Work out the finished part from the listing and answer in its coordinate system (mm). Face numbers are marked on the shaded views. A direction names the side the tool comes from. Coordinates: 2 decimals unless noted, no trailing zeros. Write each loop counter-clockwise with the first axis right and the second up, starting at its lowest first coordinate (ties: lowest second). Pieces come first, ordered by that corner, then holes. Notation, with made-up numbers: (-38.75, 59.5) - (-32.75, 59.5) arc R22 cw to (-32.75, 74.5) - close; hole circle Ø5 at (-15, 43.5). An arc over 180 degrees is marked (long way). Use a Markdown table: item, result. Add a question column.
(1) A tool of negligible diameter and unlimited length cuts with its end or side. For the marked faces 5 and 6, from which of +Z, -Z, +X, -X, +Y, -Y can it reach the whole face along a straight path? Write none if from no direction.
(2) For a pull along X with two mould halves and no side action, classify the marked faces 1, 2, 3 and 4 as released by +X, released by -X, zero draft, split by the parting line, or undercut.
(3) Find the intervals of material crossed by line 1 (X direction, y = 7.95, z = -20); line 2 (Z direction, x = 32, y = 3.2); line 3 (X direction, y = 3.4, z = 20), in increasing order. Write a range as from..to.
(4) The part is cut by section A-A, the plane z = 20. Give the vertices of the cut face in (x, y).
(5) Given pin 1 Ø6 at (x, z) = (-28.5, -5.5) entering from +Y; pin 2 Ø6.5 at (x, z) = (30.5, 20.5) entering from +Y; pin 3 Ø4 at (x, z) = (32, 20) entering from +Y, each flat-ended and moving along its own axis, determine where each tip first touches the part or whether it passes through.
(6) The part is cut by section C-C, the plane y = 35. Give the vertices of the cut face in (x, z).
(7) The part is cut by section B-B, the plane z = 2. Give the vertices of the cut face in (x, y).
(8) The part is cut by section D-D, the plane z = -20. Give the vertices of the cut face in (x, y), then the cut area to 3 significant figures.
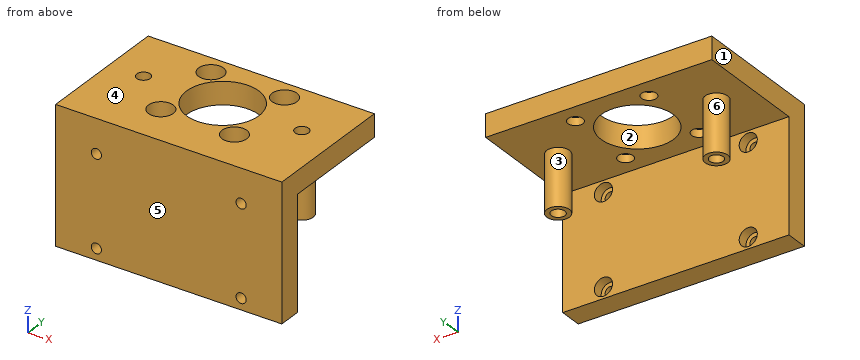
from build123d import *

# Parameters (mm, degrees)
SKETCH1_W           = 100
SKETCH1_H           = 50
BOSS_EXTRUDE1_DEPTH = 10
SKETCH2_R           = 2.25
CUT_EXTRUDE1_DEPTH  = 11
SKETCH3_R           = 4
CUT_EXTRUDE2_DEPTH  = 4.4
SKETCH4_W           = 100
SKETCH4_H           = 60
BOSS_EXTRUDE2_DEPTH = 10
SKETCH5_R           = 16
CUT_EXTRUDE3_DEPTH  = 11
SKETCH6_R           = 3.3
CUT_EXTRUDE4_DEPTH  = 11
SKETCH7_R           = 5.5
CUT_EXTRUDE5_DEPTH  = 6.6
SKETCH8_R           = 3
CUT_EXTRUDE6_DEPTH  = 11
SKETCH9_R           = 5
SKETCH9_R_2         = 3
BOSS_EXTRUDE3_DEPTH = 25


with BuildPart() as part:
    # Sketch1 → Boss-Extrude1 (new body)
    with BuildSketch(Plane(origin=(0, 0, 0), x_dir=(1, 0, 0), z_dir=(0, 1, 0))):
        Rectangle(SKETCH1_W, SKETCH1_H)
    extrude(amount=BOSS_EXTRUDE1_DEPTH)

    # Sketch2 → Cut-Extrude1 (cut, through all)
    with BuildSketch(Plane(origin=(0, 10, 0), x_dir=(1, 0, 0), z_dir=(0, 1, 0))):
        with Locations((32, 20)):
            Circle(SKETCH2_R)
        with Locations((32, -20)):
            Circle(SKETCH2_R)
        with Locations((-32, 20)):
            Circle(SKETCH2_R)
        with Locations((-32, -20)):
            Circle(SKETCH2_R)
    extrude(amount=-CUT_EXTRUDE1_DEPTH, mode=Mode.SUBTRACT)

    # Sketch3 → Cut-Extrude2 (cut)
    with BuildSketch(Plane(origin=(0, 10, 0), x_dir=(1, 0, 0), z_dir=(0, 1, 0))):
        with Locations((32, 20)):
            Circle(SKETCH3_R)
        with Locations((32, -20)):
            Circle(SKETCH3_R)
        with Locations((-32, 20)):
            Circle(SKETCH3_R)
        with Locations((-32, -20)):
            Circle(SKETCH3_R)
    extrude(amount=-CUT_EXTRUDE2_DEPTH, mode=Mode.SUBTRACT)

    # Sketch4 → Boss-Extrude2 (add)
    with BuildSketch(Plane.XY.offset(25)):
        with Locations((0, 30)):
            Rectangle(SKETCH4_W, SKETCH4_H)
    extrude(amount=BOSS_EXTRUDE2_DEPTH)

    # Sketch5 → Cut-Extrude3 (cut, through all)
    with BuildSketch(Plane(origin=(0, 0, 25), x_dir=(-1, 0, 0), z_dir=(0, 0, -1))):
        with Locations((0, 35)):
            Circle(SKETCH5_R)
    extrude(amount=-CUT_EXTRUDE3_DEPTH, mode=Mode.SUBTRACT)

    # Sketch6 → Cut-Extrude4 (cut, through all)
    with BuildSketch(Plane(origin=(0, 0, 25), x_dir=(-1, 0, 0), z_dir=(0, 0, -1))):
        with Locations((-16.25, 51.25)):
            Circle(SKETCH6_R)
        with Locations((-16.25, 18.75)):
            Circle(SKETCH6_R)
        with Locations((16.25, 18.75)):
            Circle(SKETCH6_R)
        with Locations((16.25, 51.25)):
            Circle(SKETCH6_R)
    extrude(amount=-CUT_EXTRUDE4_DEPTH, mode=Mode.SUBTRACT)

    # Sketch7 → Cut-Extrude5 (cut)
    with BuildSketch(Plane.XY.offset(35)):
        with Locations((-16.25, 51.25)):
            Circle(SKETCH7_R)
        with Locations((16.25, 51.25)):
            Circle(SKETCH7_R)
        with Locations((16.25, 18.75)):
            Circle(SKETCH7_R)
        with Locations((-16.25, 18.75)):
            Circle(SKETCH7_R)
    extrude(amount=-CUT_EXTRUDE5_DEPTH, mode=Mode.SUBTRACT)

    # Sketch8 → Cut-Extrude6 (cut, through all)
    with BuildSketch(Plane(origin=(0, 0, 25), x_dir=(-1, 0, 0), z_dir=(0, 0, -1))):
        with Locations((-35, 35)):
            Circle(SKETCH8_R)
        with Locations((35, 35)):
            Circle(SKETCH8_R)
    extrude(amount=-CUT_EXTRUDE6_DEPTH, mode=Mode.SUBTRACT)

    # Sketch9 → Boss-Extrude3 (add)
    with BuildSketch(Plane(origin=(0, 0, 25), x_dir=(-1, 0, 0), z_dir=(0, 0, -1))):
        with Locations((-35, 35)):
            Circle(SKETCH9_R)
        with Locations((-35, 35)):
            Circle(SKETCH9_R_2, mode=Mode.SUBTRACT)
        with Locations((35, 35)):
            Circle(SKETCH9_R)
        with Locations((35, 35)):
            Circle(SKETCH9_R_2, mode=Mode.SUBTRACT)
    extrude(amount=BOSS_EXTRUDE3_DEPTH)


solid = part.part
Model answer:
| question | item | result |
|---|---|---|
| 1 | face 5 | +Z, -Z, +X, -X, -Y |
| 1 | face 6 | -Z |
| 2 | face 1 | released by -X |
| 2 | face 2 | undercut |
| 2 | face 3 | undercut |
| 2 | face 4 | zero draft |
| 3 | line 1 | -50..-36, -28..28, 36..50 |
| 3 | line 2 | -25..-22.25, -17.75..17.75, 22.25..35 |
| 3 | line 3 | -50..-34.25, -29.75..29.75, 34.25..50 |
| 4 | outline | (-50, 0) - (-34.25, 0) - (-34.25, 5.6) - (-36, 5.6) - (-36, 10) - (-50, 10) - close; circle Ø10 at (-35, 35); (-29.75, 0) - (29.75, 0) - (29.75, 5.6) - (28, 5.6) - (28, 10) - (-28, 10) - (-28, 5.6) - (-29.75, 5.6) - close; circle Ø10 at (35, 35); (34.25, 0) - (50, 0) - (50, 10) - (36, 10) - (36, 5.6) - (34.25, 5.6) - close; hole circle Ø6 at (-35, 35); hole circle Ø6 at (35, 35) |
| 5 | pin 1 | y = 10 |
| 5 | pin 2 | y = 39.84 |
| 5 | pin 3 | y = 39.9 |
| 6 | outline | (-50, 25) - (-40, 25) - (-40, 0) - (-38, 0) - (-38, 35) - (-50, 35) - close; (-32, 0) - (-30, 0) - (-30, 25) - (-16, 25) - (-16, 35) - (-32, 35) - close; (16, 25) - (30, 25) - (30, 0) - (32, 0) - (32, 35) - (16, 35) - close; (38, 0) - (40, 0) - (40, 25) - (50, 25) - (50, 35) - (38, 35) - close |
| 7 | outline | (-50, 0) - (50, 0) - (50, 10) - (-50, 10) - close; circle Ø10 at (-35, 35); circle Ø10 at (35, 35); hole circle Ø6 at (-35, 35); hole circle Ø6 at (35, 35) |
| 8 | outline | (-50, 0) - (-34.25, 0) - (-34.25, 5.6) - (-36, 5.6) - (-36, 10) - (-50, 10) - close; (-29.75, 0) - (29.75, 0) - (29.75, 5.6) - (28, 5.6) - (28, 10) - (-28, 10) - (-28, 5.6) - (-29.75, 5.6) - close; (34.25, 0) - (50, 0) - (50, 10) - (36, 10) - (36, 5.6) - (34.25, 5.6) - close |
| 8 | area | 879 mm^2 |
